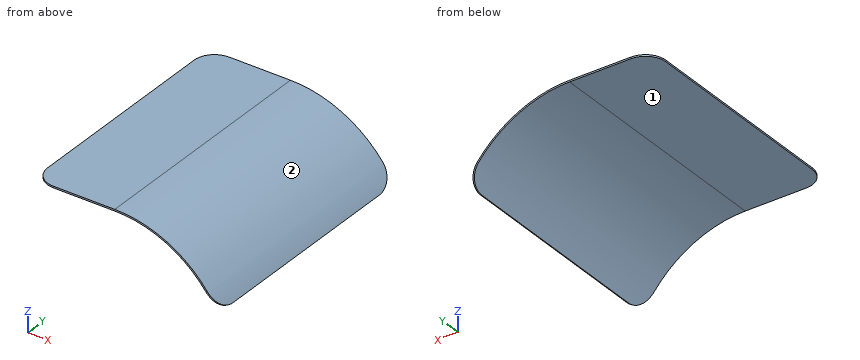
from build123d import *

# Parameters (mm, degrees)
EXTRUDE_THIN1_DEPTH = 152.4
FILLET1_START       = -34.928197123
FILLET1_DEPTH       = 36.928197123
FILLET1_START_2     = 1.736605499
FILLET1_2_DEPTH     = 83.263394501


with BuildPart() as part:
    # Sketch1 → Extrude-Thin1 (new body)
    with BuildSketch(Plane(origin=(0, 0, 0), x_dir=(1, 0, 0), z_dir=(0, 1, 0))):
        with BuildLine():
            Line((0, 0), (50.8, 0))
            ThreePointArc((50.8, 0), (87.824366436, 10.255859386), (114.294919797, 38.1))
            Line((114.294919797, 38.1), (115.191424136, 37.621945641))
            ThreePointArc((115.191424136, 37.621945641), (88.347124875, 9.384665025), (50.8, -1.016))
            Line((50.8, -1.016), (0, -1.016))
            Line((0, -1.016), (0, 0))
        make_face()
    extrude(amount=EXTRUDE_THIN1_DEPTH)

    # Fillet1: read off the stored shape, not the designer's step
    # Fillet1 outline → Fillet1 (cut)
    with BuildSketch(Plane.XY.offset(FILLET1_START)):
        with BuildLine():
            Line((0, 152.4), (0, 139.7))
            ThreePointArc((0, 139.7), (3.719743879, 148.680256121), (12.7, 152.4))
            Line((12.7, 152.4), (0, 152.4))
        make_face()
        with BuildLine():
            ThreePointArc((12.7, 0), (3.719743879, 3.719743879), (0, 12.7))
            Line((0, 12.7), (0, 0))
            Line((0, 0), (12.7, 0))
        make_face()
    extrude(amount=FILLET1_DEPTH, mode=Mode.SUBTRACT)

    # Fillet1 2 outline → Fillet1 2 (cut)
    with BuildSketch(Plane(origin=(0, 0, 0), x_dir=(0.4705259442287449, 0, -0.8823861602539153), z_dir=(0.8823861602539151, 0, 0.47052594422874505)).offset(FILLET1_START_2)):
        with BuildLine():
            Line((87.397637764, 0), (87.397637764, 12.7))
            ThreePointArc((87.397637764, 12.7), (83.677893885, 3.719743879), (74.697637764, 0))
            Line((74.697637764, 0), (87.397637764, 0))
        make_face()
        with BuildLine():
            ThreePointArc((74.697637764, 152.4), (83.677893885, 148.680256121), (87.397637764, 139.7))
            Line((87.397637764, 139.7), (87.397637764, 152.4))
            Line((87.397637764, 152.4), (74.697637764, 152.4))
        make_face()
    extrude(amount=FILLET1_2_DEPTH, mode=Mode.SUBTRACT)


solid = part.part
Could you check a few things on this model? Use its own coordinates, in mm. Face numbers are marked on the shaded views. A direction names the side the tool comes from. Coordinates: 2 decimals unless noted, no trailing zeros. Order: outer loops, then holes, each group sorted by start corner. A loop starts at its lowest first (then second) coordinate and runs counter-clockwise, first axis right, second up. Notation, with made-up numbers: (42.5, -20) - (64.5, -20) arc R11 ccw to (64.5, 0) - close; hole circle Ø9 at (86.25, 29.5). An arc over 180 degrees is marked (long way). Answer in a Markdown table with one row per item. Add a question column.
(1) Will these pins go through, and if not, where does the flat tip stop? pin 1 (1.5 mm diameter, centred on y = 63.5, z = -28, fed in from -X); pin 2 (10 mm diameter, centred on x = 67, y = 72.5, fed in from +Z); pin 3 (2 mm diameter, centred on x = 83.5, y = 66.5, fed in from +Z).
(2) If we section it at B-B, the plane x = 47.5: Please give me the cut outline in (y, z).
(3) If we section it at A-A, the plane y = 34: Please give me the cut outline in (x, z).
(4) On a 3-axis mill with a long thin cutter (end or side, diameter ignored), from which of +Z, -Z, +X, -X, +Y, -Y can I reach the whole of each face in a straight line? I mean the marked faces 1 and 2. Say none if no direction works.
(5) I need wall thicknesses on L1, parallel to Z at x = 21, y = 105.5; L2, parallel to Z at x = 54, y = 25.5; L3, parallel to X at y = 58, z = -14. Which ranges of each line are inside material? Lowest first, please.
Results are:
| question | item | result |
|---|---|---|
| 1 | pin 1 | stops at x = 107.18 |
| 1 | pin 2 | stops at z = 0.15 |
| 1 | pin 3 | stops at z = -6.23 |
| 2 | outline | (0, 0) - (152.4, 0) - (152.4, 1.02) - (0, 1.02) - close |
| 3 | outline | (0, 0) - (50.8, 0) arc R71.96 cw to (114.29, -38.1) - (115.19, -37.62) arc R72.97 ccw to (50.8, 1.02) - (0, 1.02) - close |
| 4 | face 1 | -Z, -X, +Y, -Y |
| 4 | face 2 | +Z, +X, +Y, -Y |
| 5 | L1 | z = 0 to 1.02 |
| 5 | L2 | z = -0.07 to 0.95 |
| 5 | L3 | x = 93.45 to 95.14 |
